```python
from build123d import *

# Parameters (mm, degrees)
SKETCH_1_R      = 3.5
SKETCH_1_R_2    = 2.7
EXTRUDE_1_DEPTH = 4.8
EXTRUDE_START   = -2
EXTRUDE_2_DEPTH = 2


with BuildPart() as part:
    # Sketch 1 → Extrude 1 (new body)
    with BuildSketch(Plane(origin=(0, 0, 0), x_dir=(1, 0, 0), z_dir=(0, 1, 0))):
        with Locations(Location((0, 0, 0), (0, 0, 270))):
            Circle(SKETCH_1_R)
        with Locations(Location((0, 0, 0), (0, 0, 270))):
            Circle(SKETCH_1_R_2, mode=Mode.SUBTRACT)
    extrude(amount=EXTRUDE_1_DEPTH)

    # Sketch 2 → Extrude 2 (add)
    with BuildSketch(Plane(origin=(0, 4.8, 0), x_dir=(1, 0, 0), z_dir=(0, 1, 0)).offset(EXTRUDE_START)):
        with BuildLine():
            ThreePointArc((-1.129343966, -3.312790698), (-2.707080949, -2.218493348), (-3.47009912, -0.456521739))
            Line((-3.47009912, -0.456521739), (-1.982913783, -11.760869565))
            ThreePointArc((-1.982913783, -11.760869565), (0, -13.5), (1.982913783, -11.760869565))
            Line((1.982913783, -11.760869565), (3.47009912, -0.456521739))
            ThreePointArc((3.47009912, -0.456521739), (2.707080949, -2.218493348), (1.129343966, -3.312790698))
            ThreePointArc((1.129343966, -3.312790698), (1.404282014, -3.772750509), (1.5, -4.3))
            ThreePointArc((1.5, -4.3), (1.423024947, -4.774341649), (1.2, -5.2))
            ThreePointArc((1.2, -5.2), (1.423024947, -5.625658351), (1.5, -6.1))
            ThreePointArc((1.5, -6.1), (1.423024947, -6.574341649), (1.2, -7))
            ThreePointArc((1.2, -7), (1.423024947, -7.425658351), (1.5, -7.9))
            ThreePointArc((1.5, -7.9), (1.423024947, -8.374341649), (1.2, -8.8))
            ThreePointArc((1.2, -8.8), (1.423024947, -9.225658351), (1.5, -9.7))
            ThreePointArc((1.5, -9.7), (1.423024947, -10.174341649), (1.2, -10.6))
            ThreePointArc((1.2, -10.6), (1.423024947, -11.025658351), (1.5, -11.5))
            ThreePointArc((1.5, -11.5), (-0.474341649, -12.923024947), (-1.2, -10.6))
            ThreePointArc((-1.2, -10.6), (-1.5, -9.7), (-1.2, -8.8))
            ThreePointArc((-1.2, -8.8), (-1.5, -7.9), (-1.2, -7))
            ThreePointArc((-1.2, -7), (-1.5, -6.1), (-1.2, -5.2))
            ThreePointArc((-1.2, -5.2), (-1.498949821, -4.243880178), (-1.129343966, -3.312790698))
        make_face()
    extrude(amount=EXTRUDE_2_DEPTH)


solid = part.part
```
Check sheet for the modelled part. Datum: model origin and axes. Units: mm. A direction names the side the tool comes from. Coordinates: 2 decimals unless noted, no trailing zeros. Loops run counter-clockwise (first coordinate to the right, second up) from the corner with the lowest first, then second, coordinate; pieces in that order, holes last.
1) Release check for a two-part mould opening along X. For faces 1 (the face through (2.716, 3.786, 6.188)), 2 (the face through (-1.5, 3.8, 9.7)), 3 (the face through (-1.5, 3.8, 7.9)), 4 (the face through (0, 4.8, 3)) record: released by +X, released by -X, zero draft, split by the parting line, or undercut.
2) Sectioned sample at C-C (y = 3.3). Record the boundary of the cut face in (x, z).
3) Gauge pin test, flat ends, axial feed: pin 1 (1.5 mm diameter, centred on y = 2.5, z = 7, fed in from -X); pin 2 (3.5 mm diameter, centred on x = 0, z = 11.5, fed in from -Y). Record the tip position at first contact, or that the pin passes through.
4) Sectioned sample at D-D (x = -2.5). Record the boundary of the cut face in (y, z), and give its area (3 significant figures).
5) Material ranges on probe 1 along X at (y, z) = (4.2, 0); probe 2 along Z at (x, y) = (1, 2.85); probe 3 along Z at (x, y) = (-0.25, 2.85), recorded low to high.
6) Sectioned sample at A-A (z = 0). Record the boundary of the cut face in (x, y), and give its area (3 significant figures).
7) Access from +Z, -Z, +X, -X, +Y, -Y to the whole of each face (thin tool, end or side, straight path). Record for faces 5 (the face through (-1.5, 3.8, 4.3)), 6 (the face through (-3, 0, 1)), 7 (the face through (0.154, 2.366, -3.497)).
8) Sectioned sample at B-B (x = 0). Record the boundary of the cut face in (y, z), and give its area (3 significant figures).
Check sheet entries:
1. face 1: released by +X
1. face 2: undercut
1. face 3: undercut
1. face 4: zero draft
2. outline: (-3.47, 0.46) arc R3.5 ccw (long way) to (3.47, 0.46) - (1.98, 11.76) arc R2 ccw to (-1.98, 11.76) - close; hole circle Ø5.4 at (0, 0); hole (-1.2, 5.2) arc R1.5 ccw to (-1.13, 3.31) arc R3.5 cw to (1.13, 3.31) arc R1.5 ccw to (1.2, 5.2) arc R1.5 ccw to (1.2, 7) arc R1.5 ccw to (1.2, 8.8) arc R1.5 ccw to (1.2, 10.6) arc R1.5 ccw (long way) to (-1.2, 10.6) arc R1.5 ccw to (-1.2, 8.8) arc R1.5 ccw to (-1.2, 7) arc R1.5 ccw to start
3. pin 1: stops at x = -2.7
3. pin 2: stops at y = 2.8
4. outline: (0, -2.45) - (4.8, -2.45) - (4.8, -1.02) - (0, -1.02) - close; (0, 1.02) - (4.8, 1.02) - (4.8, 7.83) - (2.8, 7.83) - (2.8, 2.45) - (0, 2.45) - close
4. area: 24.5 mm2
5. probe 1: x = -3.5 to -2.7, 2.7 to 3.5
5. probe 2: z = -3.35 to -2.51, 2.51 to 3.35, 12.62 to 13.23
5. probe 3: z = -3.49 to -2.69, 2.69 to 3.49, 12.98 to 13.48
6. outline: (-3.5, 0) - (-2.7, 0) - (-2.7, 4.8) - (-3.5, 4.8) - close; (2.7, 0) - (3.5, 0) - (3.5, 4.8) - (2.7, 4.8) - close
6. area: 7.68 mm2
7. face 5: +Y, -Y
7. face 6: +Z, -Z, +X, -X, -Y
7. face 7: -Y
8. outline: (0, -3.5) - (4.8, -3.5) - (4.8, -2.7) - (0, -2.7) - close; (0, 2.7) - (4.8, 2.7) - (4.8, 3.5) - (0, 3.5) - close; (2.8, 13) - (4.8, 13) - (4.8, 13.5) - (2.8, 13.5) - close
8. area: 8.68 mm2
